Read the model definition and answer for the solid it produces. Units are mm, in the model's axes. Face numbers are marked on the shaded views. A direction names the side the tool comes from. Coordinates: 2 decimals unless noted, no trailing zeros. Order: outer loops, then holes, each group sorted by start corner. A loop starts at its lowest first (then second) coordinate and runs counter-clockwise, first axis right, second up. Notation, with made-up numbers: (4.25, 6) - (54.25, 6) arc R19 cw to (54.25, 19) - close; hole circle Ø5 at (15, 36.25). An arc over 180 degrees is marked (long way). Use one line per item in the form item = value.
Autodesk Inventor part; units mm, degrees
ref_plane "Arbeitsebene1" through (0, 0, 9) normal (0, 0, 1) x (1, 0, 0)
ref_plane "YZ Plane" through (0, 0, 0) normal (1, 0, 0) x (0, 1, 0)
ref_plane "XZ Plane" through (0, 0, 0) normal (0, 1, 0) x (-1, 0, 0)
sketch "Skizze1" plane through (0, 0, 0) normal (0, 0, 1) x (1, 0, 0)
  circle A0 centre (0, 0) radius 2
  dimension "d0" = 4
extrude "Extrusion1" add sketch "Skizze1" along normal blind 12
sketch "Skizze2" plane through (0, 0, 12) normal (0, 0, 1) x (1, 0, 0)
  circle A0 centre (0, 0) radius 2
  line L0 (-1.9372, 0.4972) -> (1.9372, 0.4972)
extrude "Extrusion2" cut sketch "Skizze2" against normal blind 3 contours L0 A0 picked at (-0.0798, 0.9933)
ref_plane "Arbeitsebene1" through (0, 0, 9) normal (0, 0, 1) x (1, 0, 0)
sketch "Skizze3" plane through (0, 0, 9) normal (0, 0, 1) x (1, 0, 0)
  circle A0 centre (0, 0) radius 1
  arc A1 (1.9372, 0.4972) -> (-1.9372, 0.4972) centre (0, 0) ccw
  arc A2 (-1.9372, 0.4972) -> (1.9372, 0.4972) centre (0, 0) ccw
  dimension "d6" = 2
extrude "Extrusion3" cut sketch "Skizze3" against normal blind 1
properties part number "motor" material "Aluminium 6061"
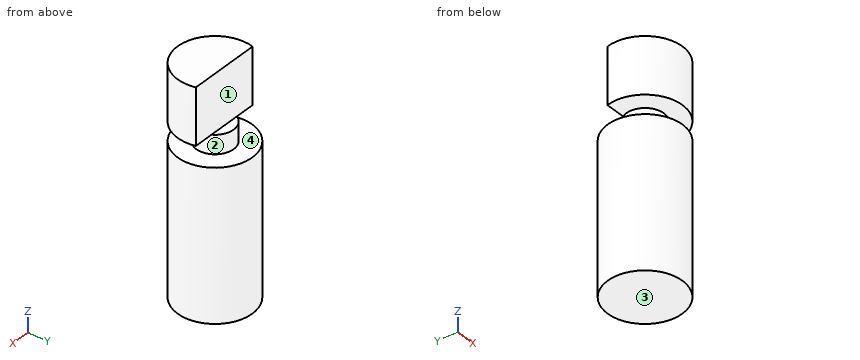
(1) Section B-B, the plane x = 0 is taken. Write down the section's boundary in (y, z).
Answer list:
outline = (-2, 0) - (2, 0) - (2, 8) - (1, 8) - (1, 9) - (0.5, 9) - (0.5, 12) - (-2, 12) - (-2, 9) - (-1, 9) - (-1, 8) - (-2, 8) - close
(2) Section D-D, the plane z = 11 is taken. Write down the section's boundary in (x, y).
Answer list:
outline = (-1.94, 0.5) arc R2 ccw (long way) to (1.94, 0.5) - close
(3) Straight lines are drawn through the part: L1, parallel to Z at x = 0.55, y = -1.65; L2, parallel to Y at x = 0.05, z = 8.25; L3, parallel to Y at x = 0.5, z = 6.75. For each, find the intervals that lie inside material, in ascending order.
Answer list:
L1 = 0 to 8, 9 to 12
L2 = -1 to 1
L3 = -1.94 to 1.94
(4) Given pin 1 Ø1 at (x, z) = (-1, 3.5) entering from -Y; pin 2 Ø0.9 at (x, z) = (1, 10.5) entering from +Y, each flat-ended and moving along its own axis, determine where each tip first touches the part or whether it passes through.
Answer list:
pin_1 = -1.94
pin_2 = 0.5
(5) Which of the six approach directions +Z, -Z, +X, -X, +Y, -Y give full straight-line access (tool end or side, diameter ignored) to the marked faces 3 and 4?
Answer list:
face_3 = -Z, +X, -X, +Y, -Y
face_4 = none
(6) The mould has two halves that part along X. Classify the marked faces 1 and 2: +X half, -X half, draft (parallel to the pull), parting line (faces both ways), or undercut.
Answer list:
face_1 = draft
face_2 = parting line
(7) Section A-A, the plane y = 0 is taken. Write down the section's boundary in (x, z), then the cut area to 3 significant figures.
Answer list:
outline = (-2, 0) - (2, 0) - (2, 8) - (1, 8) - (1, 9) - (2, 9) - (2, 12) - (-2, 12) - (-2, 9) - (-1, 9) - (-1, 8) - (-2, 8) - close
area = 46.0 mm2
(8) Section C-C, the plane z = 3.25 is taken. Write down the section's boundary in (x, y), then the cut area to 3 significant figures.
Answer list:
outline = circle Ø4 at (0, 0)
area = 12.6 mm2
